Design review of the part built by this model. Coordinates are the model's own, in mm. Face numbers are marked on the shaded views. A direction names the side the tool comes from. Round coordinates to 2 decimals unless told otherwise and drop trailing zeros. Order: outer loops, then holes, each group sorted by start corner. A loop starts at its lowest first (then second) coordinate and runs counter-clockwise, first axis right, second up. Notation, with made-up numbers: (50.5, -37) - (54.5, -37) arc R15 ccw to (54.5, -27) - close; hole circle Ø2 at (81.5, 87.25). An arc over 180 degrees is marked (long way). Answer as a JSON object with one key per item and string values. Group by question number.
from build123d import *

# Parameters (mm, degrees)
CROQUIS1_W              = 120
CROQUIS1_H              = 70
SALIENTE_EXTRUIR1_DEPTH = 60
CROQUIS2_W              = 106
CROQUIS2_H              = 56
CORTAR_EXTRUIR1_DEPTH   = 53
CROQUIS3_W              = 43
CROQUIS3_H              = 29
CORTAR_EXTRUIR2_DEPTH   = 20
CROQUIS4_W              = 21
CROQUIS4_H              = 47.698466119
SALIENTE_EXTRUIR2_DEPTH = 32
CROQUIS5_W              = 43
CROQUIS5_H              = 29
CORTAR_EXTRUIR3_DEPTH   = 16


with BuildPart() as part:
    # Croquis1 → Saliente-Extruir1 (new body)
    with BuildSketch(Plane(origin=(0, 0, 0), x_dir=(1, 0, 0), z_dir=(0, 1, 0))):
        with Locations((16.5, -1.5)):
            Rectangle(CROQUIS1_W, CROQUIS1_H)
    extrude(amount=SALIENTE_EXTRUIR1_DEPTH)

    # Croquis2 → Cortar-Extruir1 (cut)
    with BuildSketch(Plane(origin=(0, 0, 0), x_dir=(1, 0, 0), z_dir=(0, 1, 0))):
        with Locations((16.5, -1.5)):
            Rectangle(CROQUIS2_W, CROQUIS2_H)
    extrude(amount=CORTAR_EXTRUIR1_DEPTH, mode=Mode.SUBTRACT)

    # Croquis3 → Cortar-Extruir2 (cut)
    with BuildSketch(Plane.ZY.offset(43.5)):
        with Locations((-5, 38.5)):
            Rectangle(CROQUIS3_W, CROQUIS3_H)
    extrude(amount=-CORTAR_EXTRUIR2_DEPTH, mode=Mode.SUBTRACT)

    # Croquis4 → Saliente-Extruir2 (add)
    with BuildSketch(Plane.XZ.offset(-53)):
        with Locations((-26, -2.65076694)):
            Rectangle(CROQUIS4_W, CROQUIS4_H)
    extrude(amount=SALIENTE_EXTRUIR2_DEPTH)

    # Croquis5 → Cortar-Extruir3 (cut)
    with BuildSketch(Plane.ZY.offset(36.5)):
        with Locations((-5, 38.5)):
            Rectangle(CROQUIS5_W, CROQUIS5_H)
    extrude(amount=-CORTAR_EXTRUIR3_DEPTH, mode=Mode.SUBTRACT)


solid = part.part
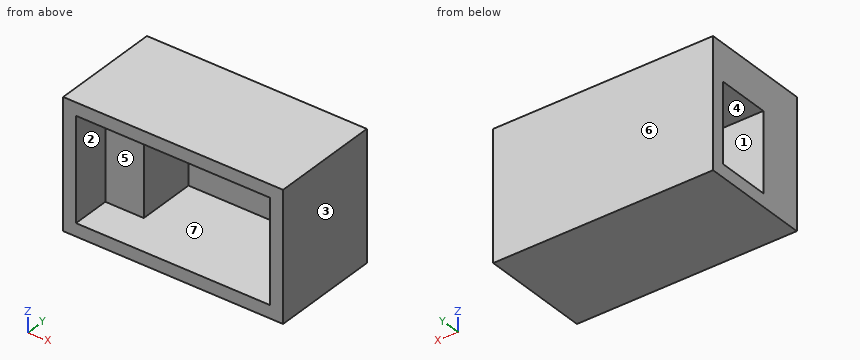
1. Mouldability with a two-part tool opening along Y and no side actions: class the marked faces 4, 5, 6 and 7 as pulls with the +Y half, pulls with the -Y half, needs draft (parallel to the pull), parting line crosses it, or undercut.
2. Take a section at A-A, the plane y = 11.5. Give the boundary of the cut face in (x, z).
3. Tool access review of the marked faces 1, 2 and 3: name each direction out of +Z, -Z, +X, -X, +Y, -Y from which nothing blocks a thin tool from reaching the whole face with its end or side.
4. Take a section at D-D, the plane x = 67.5. Give the boundary of the cut face in (y, z), then the cut area to 3 significant figures.
5. Take a section at B-B, the plane x = -28.5. Give the boundary of the cut face in (y, z), then the cut area to 3 significant figures.
6. To check wall thickness, follow line 1 (X direction, y = 41, z = -16.5); line 2 (Z direction, x = 6, y = 20); line 3 (X direction, y = 8, z = -11.5). State the ranges of each line that lie inside material, in increasing order. Write a range as from..to.
7. Take a section at C-C, the plane z = -24. Give the boundary of the cut face in (x, y), then the cut area to 3 significant figures.
8. Clearance check with flat-ended pins moving along their axes: P1, Ø6.5, axis at x = -24, z = -3.5, coming from the -Y side; P2, Ø8, axis at x = 33, z = 16.5, coming from the -Y side. State where each tip first meets the part, or that it passes through.
Response values:
{
 "1": {"face 4": "undercut", "face 5": "pulls with the -Y half", "face 6": "pulls with the +Y half", "face 7": "needs draft"},
 "2": {"outline": "(-43.5, -33.5) - (76.5, -33.5) - (76.5, 36.5) - (-43.5, 36.5) - close; hole (-36.5, -26.5) - (69.5, -26.5) - (69.5, 29.5) - (-36.5, 29.5) - close"},
 "3": {"face 1": "-X", "face 2": "-Y", "face 3": "+Z, -Z, +X, +Y, -Y"},
 "4": {"outline": "(0, -33.5) - (60, -33.5) - (60, 36.5) - (0, 36.5) - (0, 29.5) - (53, 29.5) - (53, -26.5) - (0, -26.5) - close", "area": "1,230 mm2"},
 "5": {"outline": "(0, -33.5) - (60, -33.5) - (60, 36.5) - (0, 36.5) - (0, 29.5) - (53, 29.5) - (53, 21.2) - (21, 21.2) - (21, -26.5) - (0, -26.5) - close; hole (24, -26.5) - (53, -26.5) - (53, 16.5) - (24, 16.5) - close", "area": "1,510 mm2"},
 "6": {"line 1": "-20.5..-15.5, 69.5..76.5", "line 2": "-33.5..-26.5, 29.5..36.5", "line 3": "-43.5..-36.5, 69.5..76.5"},
 "7": {"outline": "(-43.5, 0) - (-36.5, 0) - (-36.5, 21) - (-15.5, 21) - (-15.5, 53) - (69.5, 53) - (69.5, 0) - (76.5, 0) - (76.5, 60) - (-43.5, 60) - (-43.5, 53) - (-20.5, 53) - (-20.5, 24) - (-43.5, 24) - close", "area": "1,590 mm2"},
 "8": {"P1": "y = 21", "P2": "y = 53"}
}
